Input: part model. Units: mm. Frame: model coordinates. A direction names the side the tool comes from. Coordinates: 2 decimals unless noted, no trailing zeros. Write each loop counter-clockwise with the first axis right and the second up, starting at its lowest first coordinate (ties: lowest second). Pieces come first, ordered by that corner, then holes. Notation, with made-up numbers: (-30, 46.25) - (21, 46.25) arc R16 ccw to (21, 58.25) - close; hole circle Ø8 at (-20, 6.25). An arc over 180 degrees is marked (long way). Use a Markdown table: item, result. Add a question column.
Q1. Mould query, pull axis Z, two halves, no side actions, for faces 1 (the face through (-99, -9, 127)), 2 (the face through (-99, 33, 228.6)), 3 (the face through (-133, -49.268, 105)). Classes: released by +Z, released by -Z, zero draft, split by the parting line, or undercut.
Q2. Material intervals for probe 1 along Z at (x, y) = (-114, 27); probe 2 along X at (y, z) = (21.5, 147); probe 3 along X at (y, z) = (31.5, 19), sorted ascending. Write a range as from..to.
Q3. Set-up query: faces 4 (the face through (-99, 52.332, 113)), 5 (the face through (-99, 14.232, 200)), 6 (the face through (55.333, 12, 87)), 7 (the face through (-198.667, 1, 52)), 8 (the face through (-46.267, 33, 158)). Return all of +Z, -Z, +X, -X, +Y, -Y with unobstructed straight access to the full face (end or side cutting, diameter ignored); none if empty.
Q4. Section query C-C (y = 45.5). Return the cut outline in (x, z).
Q5. Section query D-D (x = -35). Return the cut outline in (y, z), then the cut area to 3 significant figures.
Q6. Pin query (flat end, axial travel): P1, Ø12, axis at x = -7, y = -6.5, coming from the -Z side. Return the tip coordinate at first contact, or that it passes through.
Q7. Section query A-A (z = 35). Return the cut outline in (x, y).
Q8. Section query B-B (x = -81). Return the cut outline in (y, z).
from build123d import *

# Parameters (mm, degrees)
F0_W     = 304.8
F0_H     = 101.6
F1_DEPTH = 127
F3_DEPTH = 101.601
F4_W     = 50.8
F4_H     = 38.1
F5_DEPTH = 101.6
F6_W     = 38.1
F6_H     = 38.1
F7_DEPTH = 101.6


with BuildPart() as f1:
    # F0 (on Top) → F1 (new body)
    with BuildSketch(Plane.XY):
        with Locations((-97.066794, 1.532109)):
            Rectangle(F0_W, F0_H)
    extrude(amount=F1_DEPTH)

    # F2 (on face) → F3 (cut, through all)
    with BuildSketch(Plane.XZ.offset(49.267891)):
        Polygon((-198.666794, 63.5), (-198.666794, 0), (4.533206, 0), (4.533206, 63.5), (4.533206, 101.6), (-198.666794, 101.6), align=None)
    extrude(amount=-F3_DEPTH, mode=Mode.SUBTRACT)

    # F4 (on face) → F5 (join)
    with BuildSketch(Plane.XY.offset(127)):
        with Locations((-224.066794, 33.282109)):
            Rectangle(F4_W, F4_H)
        with Locations((-173.266794, 33.282109)):
            Rectangle(F4_W, F4_H)
        with Locations((-20.866794, 33.282109)):
            Rectangle(F4_W, F4_H)
        with Locations((29.933206, 33.282109)):
            Rectangle(F4_W, F4_H)
    extrude(amount=F5_DEPTH)

    # F6 (on face) → F7 (join)
    with BuildSketch(Plane.YZ.offset(-147.866794)):
        with Locations((33.282109, 209.55)):
            Rectangle(F6_W, F6_H)
    extrude(amount=F7_DEPTH)


solid = f1.part
Values follow:
| question | item | result |
|---|---|---|
| 1 | face 1 | undercut |
| 1 | face 2 | released by +Z |
| 1 | face 3 | zero draft |
| 2 | probe 1 | 101.6..127, 190.5..228.6 |
| 2 | probe 2 | -249.47..-147.87, -46.27..55.33 |
| 2 | probe 3 | -249.47..-198.67, 4.53..55.33 |
| 3 | face 4 | +Z, -Z, +X, -X, +Y |
| 3 | face 5 | +Z, +X, -X, -Y |
| 3 | face 6 | +Z, -Z, +X, +Y, -Y |
| 3 | face 7 | -Z, +Y, -Y |
| 3 | face 8 | +Y, -Y |
| 4 | outline | (-249.47, 0) - (-198.67, 0) - (-198.67, 101.6) - (4.53, 101.6) - (4.53, 0) - (55.33, 0) - (55.33, 228.6) - (-249.47, 228.6) - close; hole (-147.87, 127) - (-46.27, 127) - (-46.27, 190.5) - (-147.87, 190.5) - close |
| 5 | outline | (-49.27, 101.6) - (52.33, 101.6) - (52.33, 228.6) - (14.23, 228.6) - (14.23, 127) - (-49.27, 127) - close |
| 5 | area | 6,450 mm2 |
| 6 | P1 | z = 101.6 |
| 7 | outline | (-249.47, -49.27) - (-198.67, -49.27) - (-198.67, 52.33) - (-249.47, 52.33) - close; (4.53, -49.27) - (55.33, -49.27) - (55.33, 52.33) - (4.53, 52.33) - close |
| 8 | outline | (-49.27, 101.6) - (52.33, 101.6) - (52.33, 127) - (-49.27, 127) - close; (14.23, 190.5) - (52.33, 190.5) - (52.33, 228.6) - (14.23, 228.6) - close |
